Print and shaded views of the part. All mm, measured from the part's lowest x, y and z. A direction names the side the tool comes from. Give positions to 0.01 mm unless a question says otherwise; leave off trailing zeros. Loops run counter-clockwise (first coordinate to the right, second up) from the corner with the lowest first, then second, coordinate; pieces in that order, holes last.
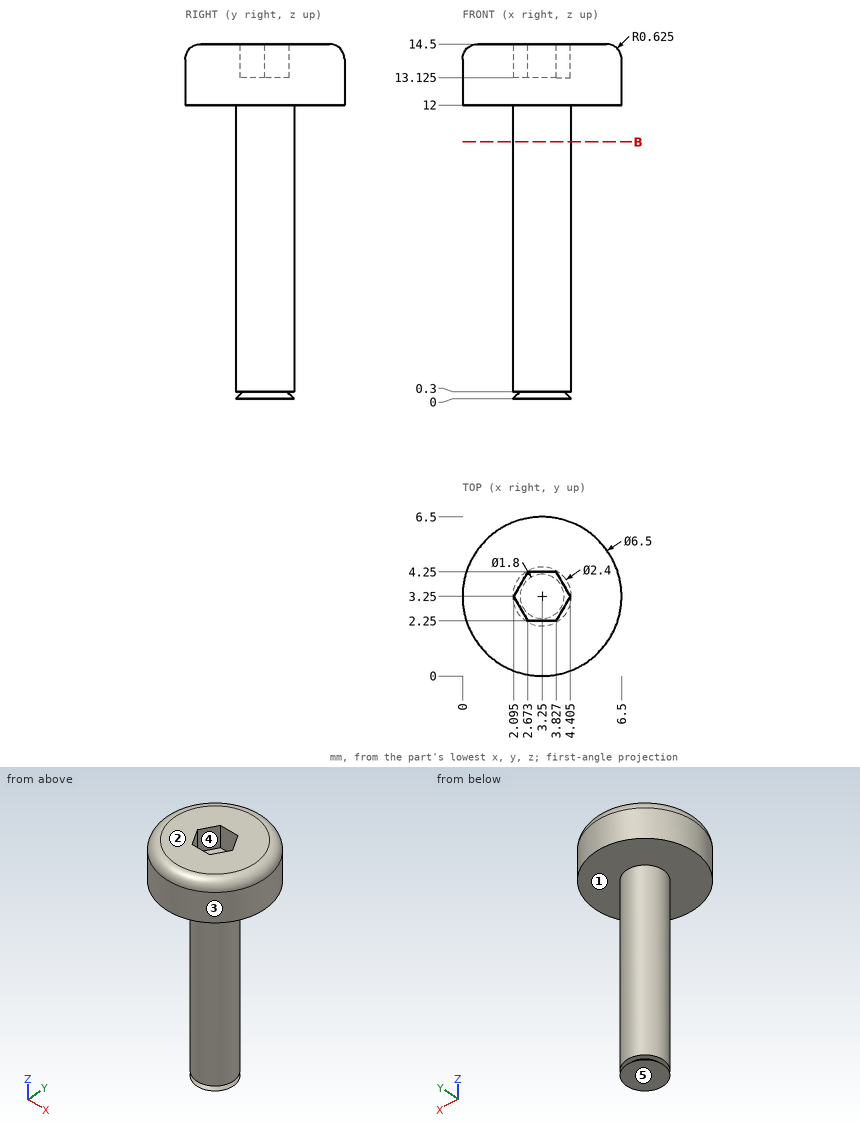
1. Pull direction X, two halves, no side cores. Call the marked faces 3, 4 and 5: released by +X, released by -X, zero draft, split by the parting line, or undercut.
Responses:
face 3: split by the parting line
face 4: undercut
face 5: zero draft
2. Saw through at B-B, the plane z = 10.5. List the corners of the cut face in (x, y).
Responses:
outline: circle Ø2.4 at (3.25, 3.25)
3. Drop flat-ended pins along their axis: pin 1 (1 mm diameter, centred on y = 1, z = 4, fed in from -X); pin 2 (1.5 mm diameter, centred on x = 2, z = 4, fed in from +Y); pin 3 (1.5 mm diameter, centred on y = 5, z = 12.5, fed in from +X). Give the stop position or say it passes through.
Responses:
pin 1: passes through
pin 2: stops at y = 4.34
pin 3: stops at x = 6.34
4. Probe line 1 along Z through (x, y) = (5.75, 2.25); line 2 along Y through (x, z) = (3.25, 6); line 3 along Z through (x, y) = (3, 3) (1 decimal). List the from-to ranges inside material, lowest first.
Responses:
line 1: z = 12 to 14.5
line 2: y = 2.05 to 4.45
line 3: z = 0 to 13.1
5. Tool access for the marked faces 1 and 2: list every direction of +Z, -Z, +X, -X, +Y, -Y with a clear straight run to the whole face (end or side of a thin tool).
Responses:
face 1: -Z
face 2: +Z, +X, -X, +Y, -Y
